```python
from build123d import *

# Parameters (mm, degrees)
BOSS_EXTRUDE1_DEPTH      = 60
SKETCH25_W               = 5.5
SKETCH25_H               = 17
BOSS_EXTRUDE3_DEPTH      = 20
FILLET1_R                = 2.3
SKETCH28_W               = 8
SKETCH28_H               = 10
CUT_EXTRUDE17_DEPTH      = 265
CUT_EXTRUDE19_DEPTH      = 165.638713704
CUT_EXTRUDE19_DEPTH_BACK = 165.638713704
SKETCH30_W               = 183.61
SKETCH30_H               = 30
CUT_EXTRUDE20_DEPTH      = 165.638713704
CUT_EXTRUDE20_DEPTH_BACK = 165.638713704
SKETCH32_W               = 3
SKETCH32_H               = 14
BOSS_EXTRUDE4_DEPTH      = 40
CUT_EXTRUDE21_DEPTH      = 90
CUT_EXTRUDE22_DEPTH      = 164.320868502
CUT_EXTRUDE22_DEPTH_BACK = 164.320868502
SKETCH39_R               = 2
CUT_EXTRUDE23_DEPTH      = 88
SKETCH40_R               = 2
CUT_EXTRUDE24_DEPTH      = 88


with BuildPart() as part:
    # Sketch1 → Boss-Extrude1 (new body)
    with BuildSketch(Plane(origin=(0, 0, 0), x_dir=(1, 0, 0), z_dir=(0, 1, 0))):
        with BuildLine():
            Line((91.805, -10), (90.252689849, -10))
            ThreePointArc((90.252689849, -10), (0, -90.805), (-90.252689849, -10))
            Line((-90.252689849, -10), (-91.805, -10))
            Line((-91.805, -10), (-91.805, 20))
            Line((-91.805, 20), (-76.805, 20))
            Line((-76.805, 20), (-76.805, 0))
            ThreePointArc((-76.805, 0), (0, -76.805), (76.805, 0))
            Line((76.805, 0), (76.805, 20))
            Line((76.805, 20), (91.805, 20))
            Line((91.805, 20), (91.805, -10))
        make_face()
    extrude(amount=-BOSS_EXTRUDE1_DEPTH)

    # Sketch25 → Boss-Extrude3 (add)
    with BuildSketch(Plane(origin=(0, -60, 0), x_dir=(-1, 0, 0), z_dir=(0, -1, 0))):
        with Locations((84.305, 5)):
            Rectangle(SKETCH25_W, SKETCH25_H)
        with Locations((-84.305, 5)):
            Rectangle(SKETCH25_W, SKETCH25_H)
    extrude(amount=BOSS_EXTRUDE3_DEPTH)

    # Fillet1
    fillet1_edges = [part.edges().sort_by_distance(p)[0] for p in [
        (84.305, -60, 3.5),
        (81.555, -60, -5),
        (87.055, -60, -5),
        (84.305, -60, -13.5),
        (-84.305, -60, 3.5),
        (-87.055, -60, -5),
        (-81.555, -60, -5),
        (-84.305, -60, -13.5),
    ]]
    fillet(fillet1_edges, radius=FILLET1_R)

    # Sketch28 → Cut-Extrude17 (cut)
    with BuildSketch(Plane(origin=(91.805, 0, 0), x_dir=(0, 0, -1), z_dir=(1, 0, 0))):
        with Locations((5, -42)):
            Rectangle(SKETCH28_W, SKETCH28_H)
    extrude(amount=-CUT_EXTRUDE17_DEPTH, mode=Mode.SUBTRACT)

    # Sketch30 → Cut-Extrude19 (cut, two sides: drawn at the far end of the back side and taken through both)
    with BuildSketch(Plane(origin=(0, 0, -20), x_dir=(-1, 0, 0), z_dir=(0, 0, -1)).offset(-CUT_EXTRUDE19_DEPTH_BACK)):
        with Locations((0, -15)):
            Rectangle(SKETCH30_W, SKETCH30_H)
    extrude(amount=CUT_EXTRUDE19_DEPTH + CUT_EXTRUDE19_DEPTH_BACK, mode=Mode.SUBTRACT)

    # Sketch32 → Cut-Extrude20 (cut, two sides: drawn at the far end of the back side and taken through both)
    with BuildSketch(Plane(origin=(0, 0, -20), x_dir=(-1, 0, 0), z_dir=(0, 0, -1)).offset(-CUT_EXTRUDE20_DEPTH_BACK)):
        with Locations((-65.13523483, -44)):
            Rectangle(SKETCH32_W, SKETCH32_H)
        with Locations((-51.773928511, -44)):
            Rectangle(SKETCH32_W, SKETCH32_H)
        with Locations((-84.305, -46)):
            Rectangle(SKETCH32_W, SKETCH32_H)
        with Locations((65.13523483, -44)):
            Rectangle(SKETCH32_W, SKETCH32_H)
        with Locations((51.773928511, -44)):
            Rectangle(SKETCH32_W, SKETCH32_H)
        with Locations((84.305, -46)):
            Rectangle(SKETCH32_W, SKETCH32_H)
    extrude(amount=CUT_EXTRUDE20_DEPTH + CUT_EXTRUDE20_DEPTH_BACK, mode=Mode.SUBTRACT)

    # Sketch33 → Boss-Extrude4 (add)
    with BuildSketch(Plane(origin=(0, -60, 0), x_dir=(-1, 0, 0), z_dir=(0, -1, 0))):
        with BuildLine():
            Line((90.252689849, -10), (76.151218145, -10))
            ThreePointArc((76.151218145, -10), (71.169996018, -28.876282513), (61.590580503, -45.886909008))
            Line((61.590580503, -45.886909008), (73.898492454, -52.768938193))
            ThreePointArc((73.898492454, -52.768938193), (84.815671791, -32.432234638), (90.252689849, -10))
        make_face()
    extrude(amount=BOSS_EXTRUDE4_DEPTH)

    # Sketch37 → Cut-Extrude21 (cut)
    with BuildSketch(Plane(origin=(0, 0, 0), x_dir=(0, 0, -1), z_dir=(1, 0, 0))):
        with BuildLine():
            Line((-0.881303102, -100), (-23.690614963, -100))
            ThreePointArc((-23.690614963, -100), (-31.684760451, -85.14357588), (-45.886909008, -76.037606625))
            Line((-45.886909008, -76.037606625), (-45.886909008, -59.917167305))
            Line((-45.886909008, -59.917167305), (-66.948234535, -59.917167305))
            Line((-66.948234535, -59.917167305), (-63.746381293, -92.441906362))
            Line((-63.746381293, -92.441906362), (-47.571757556, -115.346464391))
            Line((-47.571757556, -115.346464391), (-8.086377987, -115.346464391))
            Line((-8.086377987, -115.346464391), (-0.881303102, -100))
        make_face()
    extrude(amount=-CUT_EXTRUDE21_DEPTH, mode=Mode.SUBTRACT)

    # Sketch38 → Cut-Extrude22 (cut, two sides: drawn at the far end of the back side and taken through both)
    with BuildSketch(Plane(origin=(0, 0, 0), x_dir=(0, 0, -1), z_dir=(1, 0, 0)).offset(-CUT_EXTRUDE22_DEPTH_BACK)):
        Polygon((20, -30), (-90.805, -30), (-90.805, -60), (-10, -60), (-10, -100), (20, -100), (20, -60), align=None)
    extrude(amount=CUT_EXTRUDE22_DEPTH + CUT_EXTRUDE22_DEPTH_BACK, mode=Mode.SUBTRACT)

    # Sketch39 → Cut-Extrude23 (cut)
    with BuildSketch(Plane(origin=(0, 0, 10), x_dir=(-1, 0, 0), z_dir=(0, 0, -1))):
        with Locations((82.252689849, -87.5)):
            Circle(SKETCH39_R)
    extrude(amount=-CUT_EXTRUDE23_DEPTH, mode=Mode.SUBTRACT)

    # Sketch40 → Cut-Extrude24 (cut)
    with BuildSketch(Plane(origin=(0, -60, 0), x_dir=(1, 0, 0), z_dir=(0, 1, 0))):
        with Locations(Location((-74.590580503, -35.886909008, 0), (0, 0, 270))):
            Circle(SKETCH40_R)
    extrude(amount=-CUT_EXTRUDE24_DEPTH, mode=Mode.SUBTRACT)


solid = part.part
```
Model file for the job. Use its own axes, mm. Round coordinates to 2 decimals unless told otherwise and drop trailing zeros. Loops run counter-clockwise (first coordinate to the right, second up) from the corner with the lowest first, then second, coordinate; pieces in that order, holes last. Notation, with made-up numbers: M 21,65.25 L 74,65.25 A8 ccw 74,70.25 Z; hole C 7,44 d3. An arc over 180 degrees is marked long. Put each result on its own line as item: value. Start each with the question number.
Item 1: Drill centre lines: line 1 along X through (y, z) = (-87, 15); line 2 along Y through (x, z) = (-83.5, 15); line 3 along X through (y, z) = (-72, 19). Where is each one in solid material? Low to high.
Item 2: Mould opens along Z. For faces 1 (the face through (-87.36, -75.28, 24.78)), 2 (the face through (-75.81, -71.33, 34.3)), 3 (the face through (-79, -60, 28)), 4 (the face through (-83, -80, 10)) say: released by +Z, released by -Z, zero draft, split by the parting line, or undercut.
Item 3: Cut at B-B (y = -87.5). List the corners of the cut face in (x, z) (3 decimals), then the cut area to 3 significant figures.
Item 4: Drop flat-ended pins along their axis: P1, Ø6.5, axis at x = -82.25, y = -87.5, coming from the +Z side; P2, Ø3, axis at x = -71, y = -92, coming from the +Z side; P3, Ø8, axis at y = -91.5, z = 23.5, coming from the -X side. Give the stop position or say it passes through.
Item 5: Cut at C-C (z = 17). List the corners of the cut face in (x, y).
Item 6: Cut at D-D (y = -73). List the corners of the cut face in (x, z) (3 decimals), then the cut area to 3 significant figures.
Item 7: Cut at A-A (z = 35.5). List the corners of the cut face in (x, y).
Answer block:
1. line 1: -89.56 to -84.19, -80.32 to -75.33
1. line 2: -100 to -89.06, -85.94 to -60
1. line 3: -88.79 to -74.42
2. face 1: released by +Z
2. face 2: undercut
2. face 3: zero draft
2. face 4: released by -Z
3. outline: M -90.253,10 L -84.253,10 L -84.253,29.695 L -85.812,29.695 A90.805 ccw Z; M -80.253,10 L -76.151,10 A76.805 cw -70.832,29.695 L -80.253,29.695 Z
3. area: 206 mm2
4. P1: z = 32.54
4. P2: z = 27.53
4. P3: x = -88.69
5. outline: M -89.2,-100 L -74.9,-100 L -74.9,-60 L -89.2,-60 Z; hole C -82.25,-87.5 d4
6. outline: M -90.253,10 L -76.151,10 A76.805 cw -61.591,45.887 L -78.358,45.887 A90.805 ccw Z; hole C -74.591,35.887 d4
6. area: 527 mm2
7. outline: M -83.58,-81.62 L -76.55,-81.62 L -76.55,-60 L -83.58,-60 Z; M -72.63,-81.62 L -68.11,-81.62 L -68.11,-60 L -72.63,-60 Z
